Geometry: final body of the model. Coordinates: model frame, mm. A direction names the side the tool comes from. Round coordinates to 2 decimals unless told otherwise and drop trailing zeros. Order: outer loops, then holes, each group sorted by start corner. A loop starts at its lowest first (then second) coordinate and runs counter-clockwise, first axis right, second up. Notation, with made-up numbers: M 26,84 L 77,84 A31 cw 77,108 Z; hole C 39,53.25 d8. An arc over 180 degrees is marked long. Return JSON: item names as keys, results as strings. Group by question number.
Q1. Cut plane B-B on x = 5.5. Output: boundary loops of the cut face in (y, z).
Q2. Cut plane A-A on z = 1.9. Count the separate pieces of the cut face and the enclosed holes in it, and give its area (3 significant figures).
Q3. Contact query for flat-ended pins moving along their axis: pin 1 (0.6 mm diameter, centred on y = 0.5, z = 2, fed in from +X); pin 2 (0.7 mm diameter, centred on x = 6, z = 2, fed in from +Y); pin 3 (0.8 mm diameter, centred on x = -4, z = 2, fed in from -Y). Output: stop coordinate, or through.
Q4. Ray query, probe 1 along Z at (x, y) = (-3.5, -1); probe 2 along Y at (x, z) = (10, 0.45); probe 3 along Y at (x, z) = (9.25, 0.4). Return the intervals inside material, ascending.
Q5. Access query for faces 1 (the face through (7.377, -1.843, 1.955)), 2 (the face through (1, 0, 2.3)). Directions: +Z, -Z, +X, -X, +Y, -Y. A direction counts if a zero-diameter tool reaches every point of the face in a straight line with its end or side. Return the directions, or none.
Q6. Mould query, pull axis Y, two halves, no side actions, for faces 3 (the face through (-7, 0, 1.6)), 4 (the face through (-2.53, -11.37, 1.13)), 5 (the face through (7, 1, 2.3)). Classes: released by +Y, released by -Y, zero draft, split by the parting line, or undercut.
Q7. Cut plane C-C on z = 0.6. Output: boundary loops of the cut face in (x, y), and give its area (3 significant figures).
Q8. Cut plane D-D on y = -8. Output: boundary loops of the cut face in (x, z).
```python
from build123d import *

# Parameters (mm, degrees)
F0_R     = 11.65
F1_DEPTH = 2.3
F3_DEPTH = 0.7


with BuildPart() as f1:
    # F0 (on Top) → F1 (new body)
    with BuildSketch(Plane.XY):
        Circle(F0_R)
    extrude(amount=F1_DEPTH)

    # F2 (on face) → F3 (cut)
    with BuildSketch(Plane.XY.offset(2.3)):
        with BuildLine():
            Line((-9.2821657193, 2.94921875), (-9.2821657193, 0))
            Line((-9.2821657193, 0), (-8.1577947596, 0))
            add(Edge.make_bspline(
                [(-8.2326865526, 1.6666666667), (-8.1704547679, 0.5330109879), (-8.1577947596, 0)],
                knots=[0, 0, 0, 0.7965668448, 0.7965668448, 0.7965668448], degree=2))
            Line((-8.2326865526, 1.6666666667), (-8.1962282193, 1.6666666667))
            Line((-8.1962282193, 1.6666666667), (-7.6846954812, 0))
            Line((-7.6846954812, 0), (-6.6522663233, 0))
            Line((-6.6522663233, 0), (-7.5647178026, 2.94921875))
            Line((-7.5647178026, 2.94921875), (-9.2821657193, 2.94921875))
        make_face()
        with BuildLine():
            Line((-8.1577947596, 0), (-9.2821657193, 0))
            Line((-9.2821657193, 0), (-9.2821657193, -3))
            Line((-9.2821657193, -3), (-8.1545615526, -3))
            Line((-8.1545615526, -3), (-8.1545615526, -0.2330729167))
            add(Edge.make_bspline(
                [(-8.1577947596, 0), (-8.1545615526, -0.1361243036), (-8.1545615526, -0.2330729167)],
                knots=[0.7965668448, 0.7965668448, 0.7965668448, 1, 1, 1], degree=2))
        make_face()
        Polygon((-5.6076865526, -3), (-4.6199839255, 0), (-5.607097373, 0), (-6.132426136, -1.6002604167), (-6.1571657193, -1.6002604167), (-6.6522663233, 0), (-7.6846954812, 0), (-6.7639365526, -3), align=None)
        with BuildLine():
            Line((-4.0973563741, 0), (-2.9227907193, 0))
            Line((-2.9227907193, 0), (-2.9227907193, 2.94921875))
            Line((-2.9227907193, 2.94921875), (-4.6389365526, 2.94921875))
            Line((-4.6389365526, 2.94921875), (-5.607097373, 0))
            Line((-5.607097373, 0), (-4.6199839255, 0))
            Line((-4.6199839255, 0), (-4.073832386, 1.6588541667))
            Line((-4.073832386, 1.6588541667), (-4.0373740526, 1.6588541667))
            add(Edge.make_bspline(
                [(-4.0920615526, 0.2760416667), (-4.085551136, 0.5364583333), (-4.0373740526, 1.6588541667)],
                knots=[0, 0, 0, 1, 1, 1], degree=2))
            add(Edge.make_bspline(
                [(-4.0973563741, 0), (-4.0957587805, 0.1281525523), (-4.0920615526, 0.2760416667)],
                knots=[0.432105801, 0.432105801, 0.432105801, 1, 1, 1], degree=2))
        make_face()
        with BuildLine():
            Line((-2.9227907193, -3), (-2.9227907193, 0))
            Line((-2.9227907193, 0), (-4.0973563741, 0))
            add(Edge.make_bspline(
                [(-4.0985719693, -0.18359375), (-4.0985719693, -0.0975101725), (-4.0973563741, 0)],
                knots=[0, 0, 0, 0.432105801, 0.432105801, 0.432105801], degree=2))
            Line((-4.0985719693, -0.18359375), (-4.0985719693, -3))
            Line((-4.0985719693, -3), (-2.9227907193, -3))
        make_face()
        Polygon((-1.425394886, 0), (-0.163676136, 0), (-0.163676136, 1.9153645833), (0, 1.9153645833), (0, 2.94921875), (-1.425394886, 2.94921875), align=None)
        with BuildLine():
            Line((-0.163676136, -1.9583333333), (-0.163676136, 0))
            Line((-0.163676136, 0), (-1.425394886, 0))
            Line((-1.425394886, 0), (-1.425394886, -3))
            Line((-1.425394886, -3), (0.2595009474, -3))
            add(Edge.make_bspline(
                [(2.674214489, -2.21875), (1.8376259474, -3), (0.2595009474, -3)],
                knots=[0, 0, 0, 1, 1, 1], degree=2))
            add(Edge.make_bspline(
                [(3.5108030307, 0.03125), (3.5108030307, -1.4375), (2.674214489, -2.21875)],
                knots=[0, 0, 0, 1, 1, 1], degree=2))
            add(Edge.make_bspline(
                [(2.7048134474, 2.1803385417), (3.5108030307, 1.4114583333), (3.5108030307, 0.03125)],
                knots=[0, 0, 0, 1, 1, 1], degree=2))
            add(Edge.make_bspline(
                [(0.441792614, 2.94921875), (1.898823864, 2.94921875), (2.7048134474, 2.1803385417)],
                knots=[0, 0, 0, 1, 1, 1], degree=2))
            Line((0.441792614, 2.94921875), (0, 2.94921875))
            Line((0, 2.94921875), (0, 1.9153645833))
            Line((0, 1.9153645833), (0.5068967807, 1.9153645833))
            add(Edge.make_bspline(
                [(2.199605114, -0.0013020833), (2.199605114, 1.9153645833), (0.5068967807, 1.9153645833)],
                knots=[0, 0, 0, 1, 1, 1], degree=2))
            add(Edge.make_bspline(
                [(0.3766884474, -1.9583333333), (2.199605114, -1.9583333333), (2.199605114, -0.0013020833)],
                knots=[0, 0, 0, 1, 1, 1], degree=2))
            Line((0.3766884474, -1.9583333333), (-0.163676136, -1.9583333333))
        make_face()
        with BuildLine():
            Line((6.0055946974, -3), (6.0055946974, -0.7174479167))
            Line((6.0055946974, -0.7174479167), (6.676167614, -0.7174479167))
            Line((6.676167614, -0.7174479167), (8.0967405307, -3))
            Line((8.0967405307, -3), (9.496480114, -3))
            add(Edge.make_bspline(
                [(7.746480114, -0.4075520833), (9.090230114, -2.4140625), (9.496480114, -3)],
                knots=[0, 0, 0, 1, 1, 1], degree=2))
            add(Edge.make_bspline(
                [(8.564839489, 0.2330729167), (8.2764280307, -0.17578125), (7.746480114, -0.4075520833)],
                knots=[0, 0, 0, 1, 1, 1], degree=2))
            add(Edge.make_bspline(
                [(8.8532509474, 1.1666666667), (8.8532509474, 0.6419270833), (8.564839489, 0.2330729167)],
                knots=[0, 0, 0, 1, 1, 1], degree=2))
            add(Edge.make_bspline(
                [(8.271870739, 2.5078125), (8.8532509474, 2.06640625), (8.8532509474, 1.1666666667)],
                knots=[0, 0, 0, 1, 1, 1], degree=2))
            add(Edge.make_bspline(
                [(6.476948864, 2.94921875), (7.6904905307, 2.94921875), (8.271870739, 2.5078125)],
                knots=[0, 0, 0, 1, 1, 1], degree=2))
            Line((6.476948864, 2.94921875), (4.7438759474, 2.94921875))
            Line((4.7438759474, 2.94921875), (4.7438759474, -3))
            Line((4.7438759474, -3), (6.0055946974, -3))
        make_face()
        with BuildLine():
            Line((6.4118446974, 0.30859375), (6.0055946974, 0.30859375))
            Line((6.0055946974, 0.30859375), (6.0055946974, 1.9153645833))
            Line((6.0055946974, 1.9153645833), (6.3884071974, 1.9153645833))
            add(Edge.make_bspline(
                [(7.2887978224, 1.736328125), (6.9977821974, 1.9153645833), (6.3884071974, 1.9153645833)],
                knots=[0, 0, 0, 1, 1, 1], degree=2))
            add(Edge.make_bspline(
                [(7.5798134474, 1.1341145833), (7.5798134474, 1.5572916667), (7.2887978224, 1.736328125)],
                knots=[0, 0, 0, 1, 1, 1], degree=2))
            add(Edge.make_bspline(
                [(7.295308239, 0.5078125), (7.5798134474, 0.70703125), (7.5798134474, 1.1341145833)],
                knots=[0, 0, 0, 1, 1, 1], degree=2))
            add(Edge.make_bspline(
                [(6.4118446974, 0.30859375), (7.0108030307, 0.30859375), (7.295308239, 0.5078125)],
                knots=[0, 0, 0, 1, 1, 1], degree=2))
        make_face(mode=Mode.SUBTRACT)
    extrude(amount=-F3_DEPTH, mode=Mode.SUBTRACT)


solid = f1.part
```
Result sheet:
{
 "1": {"outline": "M -10.27,0 L 10.27,0 L 10.27,2.3 L 2.95,2.3 L 2.95,1.6 L -3,1.6 L -3,2.3 L -10.27,2.3 Z"},
 "2": {"separate pieces": "3", "enclosed holes": "3", "area": "367 mm²"},
 "3": {"pin 1": "stops at x = 11.65", "pin 2": "stops at y = 10.19", "pin 3": "stops at y = -11.08"},
 "4": {"probe 1": "z = 0 to 1.6", "probe 2": "y = -5.98 to 5.98", "probe 3": "y = -7.08 to 7.08"},
 "5": {"face 1": "+Z", "face 2": "+Z, +X, -X, +Y, -Y"},
 "6": {"face 3": "undercut", "face 4": "split by the parting line", "face 5": "zero draft"},
 "7": {"outline": "C 0,0 d23.3", "area": "426 mm²"},
 "8": {"outline": "M -8.47,0 L 8.47,0 L 8.47,2.3 L -8.47,2.3 Z"}
}
